from build123d import *

# Parameters (mm, degrees)
EXTRUDE001_DEPTH = 3
SKETCH_W         = 12.96
SKETCH_H         = 14.18
SKETCH_R         = 0.25
SKETCH_R_2       = 1.65
EXTRUDE_DEPTH    = 2


with BuildPart() as obj1:
    # Sketch001 → Extrude001 (new body)
    with BuildSketch(Plane.XY):
        Polygon((10.18, 14.18), (10.18, 8.98), (2.78, 8.98), (2.78, 14.18), (6.48, 14.18), align=None)
    extrude(amount=EXTRUDE001_DEPTH)


with BuildPart() as obj1_1:
    # Extrude001 placement: moved
    add(obj1.part.moved(Location((0, 0, 2))))


with BuildPart() as obj2:
    # Sketch → Extrude (new body)
    with BuildSketch(Plane.XY):
        with Locations((6.48, 7.09)):
            Rectangle(SKETCH_W, SKETCH_H)
        with Locations((1, 1)):
            Circle(SKETCH_R, mode=Mode.SUBTRACT)
        with Locations((3.74, 1)):
            Circle(SKETCH_R, mode=Mode.SUBTRACT)
        with Locations((6.48, 1)):
            Circle(SKETCH_R, mode=Mode.SUBTRACT)
        with Locations((9.22, 1)):
            Circle(SKETCH_R, mode=Mode.SUBTRACT)
        with Locations((11.96, 1)):
            Circle(SKETCH_R, mode=Mode.SUBTRACT)
        with Locations((2.15, 7.435)):
            Circle(SKETCH_R_2, mode=Mode.SUBTRACT)
        with Locations((10.81, 7.435)):
            Circle(SKETCH_R_2, mode=Mode.SUBTRACT)
    extrude(amount=EXTRUDE_DEPTH)

    # Fusion: union obj1
    add(obj1_1.part)


with BuildPart() as obj2_1:
    # Fusion placement: moved
    add(obj2.part.moved(Location((-20, 0, 0))))


solid = obj2_1.part
Input: part model. Units: mm. Frame: model coordinates. A direction names the side the tool comes from. Coordinates: 2 decimals unless noted, no trailing zeros. Loops run counter-clockwise (first coordinate to the right, second up) from the corner with the lowest first, then second, coordinate; pieces in that order, holes last. Notation, with made-up numbers: (64, -5) -> (69, -5) arc R10 ccw to (69, 11) -> close; hole circle Ø4 at (-14, 13.25). An arc over 180 degrees is marked (long way). Write item = value, one per line. Start each with the question number.
Item 1: Cut plane B-B, the plane x = -13.52. Return loops of the section in (y, z), plus the area to 3 significant figures.
Item 2: Reachability of faces 1 (the face through (-13, 8.98, 3)), 2 (the face through (-9.82, 12, 3)), 3 (the face through (-16.276, 7.931, 0.986)), 4 (the face through (-14, 14.18, 2)), 5 (the face through (-17.22, 12, 3)) from +Z, -Z, +X, -X, +Y, -Y: full face, straight path, thin tool, end or side. Return the list, or none.
Item 3: Material intervals for line 1 (Y direction, x = -13.52, z = 1.05); line 2 (Y direction, x = -8.04, z = 1.2); line 3 (Y direction, x = -9.19, z = 1.2) (3 decimals), sorted ascending.
Item 4: Cut plane A-A, the plane y = 1. Return loops of the section in (x, z), plus the area to 3 significant figures.
Item 5: First-contact query: P1, Ø5, axis at x = -10, y = 3.5, coming from the -Z side; P2, Ø4, axis at x = -16.5, y = 5, coming from the +Z side; P3, Ø2.5, axis at x = -9.19, y = 7.435, coming from the -Z side; P4, Ø0.9, axis at x = -13, z = 3, coming from the -Y side. Flat tips, straight axial feed; report the tip coordinate or a pass-through.
Item 6: Cut plane C-C, the plane z = 1.75. Return loops of the section in (x, y) (3 decimals), plus the area to 3 significant figures.
Item 7: Cut plane D-D, the plane y = 11.25. Return loops of the section in (x, z), plus the area to 3 significant figures.
Ans:
q1.outline = (0, 0) -> (0.75, 0) -> (0.75, 2) -> (0, 2) -> close; (1.25, 0) -> (14.18, 0) -> (14.18, 5) -> (8.98, 5) -> (8.98, 2) -> (1.25, 2) -> close
q1.area = 43.0 mm²
q2.face_1 = +Z, +X, -X, -Y
q2.face_2 = +Z, +X, +Y, -Y
q2.face_3 = +Z, -Z
q2.face_4 = +Z, -Z, +X, -X, +Y
q2.face_5 = +Z, -X, +Y, -Y
q3.line_1 = 0 to 0.75, 1.25 to 14.18
q3.line_2 = 0 to 0.75, 1.25 to 6.25, 8.62 to 14.18
q3.line_3 = 0 to 5.785, 9.085 to 14.18
q4.outline = (-20, 0) -> (-19.25, 0) -> (-19.25, 2) -> (-20, 2) -> close; (-18.75, 0) -> (-16.51, 0) -> (-16.51, 2) -> (-18.75, 2) -> close; (-16.01, 0) -> (-13.77, 0) -> (-13.77, 2) -> (-16.01, 2) -> close; (-13.27, 0) -> (-11.03, 0) -> (-11.03, 2) -> (-13.27, 2) -> close; (-10.53, 0) -> (-8.29, 0) -> (-8.29, 2) -> (-10.53, 2) -> close; (-7.79, 0) -> (-7.04, 0) -> (-7.04, 2) -> (-7.79, 2) -> close
q4.area = 20.9 mm²
q5.P1 = 0
q5.P2 = 2
q5.P3 = through
q5.P4 = 8.98
q6.outline = (-20, 0) -> (-7.04, 0) -> (-7.04, 14.18) -> (-20, 14.18) -> close; hole circle Ø3.3 at (-17.85, 7.435); hole circle Ø0.5 at (-19, 1); hole circle Ø0.5 at (-16.26, 1); hole circle Ø0.5 at (-13.52, 1); hole circle Ø0.5 at (-10.78, 1); hole circle Ø3.3 at (-9.19, 7.435); hole circle Ø0.5 at (-8.04, 1)
q6.area = 166 mm²
q7.outline = (-20, 0) -> (-7.04, 0) -> (-7.04, 2) -> (-9.82, 2) -> (-9.82, 5) -> (-17.22, 5) -> (-17.22, 2) -> (-20, 2) -> close
q7.area = 48.1 mm²
